from build123d import *
from OCP.BRepFilletAPI import BRepFilletAPI_MakeChamfer

# Parameters (mm, degrees)
ESQUISSE1_W             = 20.32
ESQUISSE1_H             = 13.2
BOSS_EXTRU_1_DEPTH      = 6
ESQUISSE2_W             = 18.32
ESQUISSE2_H             = 11.2
ENL_V_MAT_EXTRU_1_DEPTH = 5
ESQUISSE3_W             = 5
ESQUISSE3_H             = 1
ENL_V_MAT_EXTRU_2_DEPTH = 5
ESQUISSE4_W             = 15.32
ESQUISSE4_H             = 8.2
ENL_V_MAT_EXTRU_3_DEPTH = 25.741511676
ESQUISSE6_W             = 1
ESQUISSE6_H             = 11.2
ENL_V_MAT_EXTRU_4_DEPTH = 4.75
ESQUISSE7_W             = 30
ESQUISSE7_H             = 13.2
BOSS_EXTRU_2_DEPTH      = 1.25
ESQUISSE8_W             = 1.25
ESQUISSE8_H             = 13.2
BOSS_EXTRU_3_DEPTH      = 8
ESQUISSE9_W             = 9.25
ESQUISSE9_H             = 1.25
BOSS_EXTRU_4_DEPTH      = 6
CHANFREIN1_SIZE         = 2
CHANFREIN1_SIZE_2       = 3.464101615
ESQUISSE10_W            = 28.75
ESQUISSE10_H            = 1
BOSS_EXTRU_5_DEPTH      = 2
CHANFREIN2_SIZE         = 2
CHANFREIN2_SIZE2        = 3.464101615
ESQUISSE11_W            = 21
ESQUISSE11_H            = 1.433492253
ENL_V_MAT_EXTRU_5_DEPTH = 2
ESQUISSE12_W            = 0.8
ESQUISSE12_H            = 9.25
ENL_V_MAT_EXTRU_6_DEPTH = 2
CONG_1_R                = 1.5


with BuildPart() as part:
    # Esquisse1 → Boss.-Extru.1 (new body)
    with BuildSketch(Plane.XY):
        with Locations((10.16, 6.6)):
            Rectangle(ESQUISSE1_W, ESQUISSE1_H)
    extrude(amount=BOSS_EXTRU_1_DEPTH)

    # Esquisse2 → Enlèv. mat.-Extru.1 (cut)
    with BuildSketch(Plane.XY.offset(6)):
        with Locations((10.16, 6.6)):
            Rectangle(ESQUISSE2_W, ESQUISSE2_H)
    extrude(amount=-ENL_V_MAT_EXTRU_1_DEPTH, mode=Mode.SUBTRACT)

    # Esquisse3 → Enlèv. mat.-Extru.2 (cut)
    with BuildSketch(Plane.XY.offset(6)):
        with Locations((3.5, 12.7)):
            Rectangle(ESQUISSE3_W, ESQUISSE3_H)
    extrude(amount=-ENL_V_MAT_EXTRU_2_DEPTH, mode=Mode.SUBTRACT)

    # Esquisse4 → Enlèv. mat.-Extru.3 (cut, through all)
    with BuildSketch(Plane.XY.offset(1)):
        with Locations((10.16, 6.6)):
            Rectangle(ESQUISSE4_W, ESQUISSE4_H)
    extrude(amount=-ENL_V_MAT_EXTRU_3_DEPTH, mode=Mode.SUBTRACT)

    # Esquisse6 → Enlèv. mat.-Extru.4 (cut)
    with BuildSketch(Plane.XY.offset(6)):
        with Locations((19.82, 6.6)):
            Rectangle(ESQUISSE6_W, ESQUISSE6_H)
    extrude(amount=-ENL_V_MAT_EXTRU_4_DEPTH, mode=Mode.SUBTRACT)

    # Esquisse7 → Boss.-Extru.2 (add)
    with BuildSketch(Plane(origin=(0, 0, 0), x_dir=(-1, 0, 0), z_dir=(0, 0, -1))):
        with Locations((-35.32, 6.6)):
            Rectangle(ESQUISSE7_W, ESQUISSE7_H)
    extrude(amount=-BOSS_EXTRU_2_DEPTH)

    # Esquisse8 → Boss.-Extru.3 (add)
    with BuildSketch(Plane.XY.offset(1.25)):
        with Locations((49.695, 6.6)):
            Rectangle(ESQUISSE8_W, ESQUISSE8_H)
    extrude(amount=BOSS_EXTRU_3_DEPTH)

    # Esquisse9 → Boss.-Extru.4 (add)
    with BuildSketch(Plane(origin=(50.32, 0, 0), x_dir=(0, 0, -1), z_dir=(1, 0, 0))):
        with Locations((-4.625, 11.375)):
            Rectangle(ESQUISSE9_W, ESQUISSE9_H)
        with Locations((-4.625, 1.825)):
            Rectangle(ESQUISSE9_W, ESQUISSE9_H)
    extrude(amount=BOSS_EXTRU_4_DEPTH)

    # Chanfrein1
    # the kernel refuses this chamfer: 3.464101615, 2 mm, written as the material it adds along each edge
    with BuildSketch(Plane(origin=(50.32, 12, 9.25), x_dir=(0, 1, 0), z_dir=(0, 0, -1))) as chanfrein1_piece_1_section:
        Polygon((CHANFREIN1_SIZE, 0), (0, CHANFREIN1_SIZE_2), (0, 0), align=None)
    chanfrein1_piece_1 = extrude(amount=9.25, mode=Mode.PRIVATE)
    chanfrein1_piece_1 = split(chanfrein1_piece_1, bisect_by=Plane(origin=(50.32, 13.2, 9.25), z_dir=(0, -1, 0)), keep=Keep.TOP, mode=Mode.PRIVATE)
    add(chanfrein1_piece_1)
    with BuildSketch(Plane(origin=(50.32, 1.2, 0), x_dir=(0, -1, 0), z_dir=(0, 0, 1))) as chanfrein1_piece_2_section:
        Polygon((CHANFREIN1_SIZE, 0), (0, CHANFREIN1_SIZE_2), (0, 0), align=None)
    chanfrein1_piece_2 = extrude(amount=9.25, mode=Mode.PRIVATE)
    chanfrein1_piece_2 = split(chanfrein1_piece_2, bisect_by=Plane(origin=(50.32, 0, 0), z_dir=(0, 1, 0)), keep=Keep.TOP, mode=Mode.PRIVATE)
    add(chanfrein1_piece_2)

    # Esquisse10 → Boss.-Extru.5 (add)
    with BuildSketch(Plane.XY.offset(1.25)):
        with Locations((34.695, 12.7)):
            Rectangle(ESQUISSE10_W, ESQUISSE10_H)
        with Locations((34.695, 0.5)):
            Rectangle(ESQUISSE10_W, ESQUISSE10_H)
    extrude(amount=BOSS_EXTRU_5_DEPTH)

    # Chanfrein2: one chamfer whose edges measure the first distance from different faces: ONE call of the kernel's chamfer builder (chamfer() names one face for all edges)
    chanfrein2_edges_1 = [part.edges().sort_by_distance(p)[0] for p in [
        (20.32, 12.7, 3.25),
    ]]
    chanfrein2_side_1 = [part.faces().sort_by_distance(p)[0] for p in [
        (20.32, 12.7, 4.625),
    ]]
    chanfrein2_edges_2 = [part.edges().sort_by_distance(p)[0] for p in [
        (49.07, 12.7, 3.25),
        (49.07, 0.5, 3.25),
    ]]
    chanfrein2_side_2 = [part.faces().sort_by_distance(p)[0] for p in [
        (49.07, 6.6, 5.368110236),
    ]]
    chanfrein2_edges_3 = [part.edges().sort_by_distance(p)[0] for p in [
        (20.32, 0.5, 3.25),
    ]]
    chanfrein2_side_3 = [part.faces().sort_by_distance(p)[0] for p in [
        (20.32, 0.5, 4.625),
    ]]
    chanfrein2 = BRepFilletAPI_MakeChamfer(part.part.solid().wrapped)
    for e in chanfrein2_edges_1:
        chanfrein2.Add(CHANFREIN2_SIZE, CHANFREIN2_SIZE2, e.wrapped, chanfrein2_side_1[0].wrapped)  # the first distance lies on this face
    for e in chanfrein2_edges_2:
        chanfrein2.Add(CHANFREIN2_SIZE, CHANFREIN2_SIZE2, e.wrapped, chanfrein2_side_2[0].wrapped)  # the first distance lies on this face
    for e in chanfrein2_edges_3:
        chanfrein2.Add(CHANFREIN2_SIZE, CHANFREIN2_SIZE2, e.wrapped, chanfrein2_side_3[0].wrapped)  # the first distance lies on this face
    add(Compound.cast(chanfrein2.Shape()), mode=Mode.REPLACE)

    # Esquisse11 → Enlèv. mat.-Extru.5 (cut)
    with BuildSketch(Plane.XY.offset(1.25)):
        with Locations((35.07, 9.983253874)):
            Rectangle(ESQUISSE11_W, ESQUISSE11_H)
        with Locations((35.07, 6.683253873)):
            Rectangle(ESQUISSE11_W, ESQUISSE11_H)
        with Locations((35.07, 3.383253874)):
            Rectangle(ESQUISSE11_W, ESQUISSE11_H)
    extrude(amount=-ENL_V_MAT_EXTRU_5_DEPTH, mode=Mode.SUBTRACT)

    # Esquisse12 → Enlèv. mat.-Extru.6 (cut)
    with BuildSketch(Plane(origin=(0, 1.2, 0), x_dir=(-1, 0, 0), z_dir=(0, -1, 0))):
        with Locations((-55.92, -4.625)):
            Rectangle(ESQUISSE12_W, ESQUISSE12_H)
    extrude(amount=-ENL_V_MAT_EXTRU_6_DEPTH, mode=Mode.SUBTRACT)

    # Congé1
    # the kernel refuses this fillet: 1.5 mm, written as the material it adds along each edge
    with BuildSketch(Plane(origin=(1, 1, 1), x_dir=(0, 0, 1), z_dir=(0, 1, 0))) as cong_1_piece_1:
        with BuildLine():
            CenterArc((CONG_1_R, CONG_1_R), CONG_1_R, 180, 90)
            Line((0, CONG_1_R), (0, 0))
            Line((0, 0), (CONG_1_R, 0))
        make_face()
    extrude(amount=12.2)
    with BuildSketch(Plane(origin=(6, 12.2, 1), x_dir=(-1, 0, 0), z_dir=(0, 1, 0))) as cong_1_piece_2:
        with BuildLine():
            CenterArc((CONG_1_R, CONG_1_R), CONG_1_R, 180, 90)
            Line((0, CONG_1_R), (0, 0))
            Line((0, 0), (CONG_1_R, 0))
        make_face()
    extrude(amount=1)
    # the kernel refuses this fillet: 1.5 mm, written as the material it takes off along each edge
    with BuildSketch(Plane(origin=(20.32, -3.247595264, 6), x_dir=(-1, 0, 0), z_dir=(0, 1, 0)), Plane(origin=(20.32, 8.952404736, 6), x_dir=(-1, 0, 0), z_dir=(0, 1, 0))) as cong_1_2_piece_1:
        with BuildLine():
            CenterArc((1.299038106, -1.5), CONG_1_R, 90, 60)
            Line((0, -0.75), (0, 0))
            Line((0, 0), (1.299038106, 0))
        make_face()
    extrude(amount=7.495190528, mode=Mode.SUBTRACT)
    with BuildSketch(Plane(origin=(19.32, 1, 1.25), x_dir=(1, 0, 0), z_dir=(0, 1, 0))) as cong_1_2_piece_2:
        with BuildLine():
            CenterArc((0.829156198, 1.5), CONG_1_R, 236.442690238, 33.557309762)
            Line((0, 0.25), (0, 0))
            Line((0, 0), (0.829156198, 0))
        make_face()
    extrude(amount=11.2, mode=Mode.SUBTRACT)
    with BuildSketch(Plane(origin=(6, 8.45, 6), x_dir=(0, 0, -1), z_dir=(0, 1, 0))) as cong_1_2_piece_3:
        with BuildLine():
            CenterArc((CONG_1_R, -CONG_1_R), CONG_1_R, 90, 90)
            Line((0, -CONG_1_R), (0, 0))
            Line((0, 0), (CONG_1_R, 0))
        make_face()
    extrude(amount=8.5, mode=Mode.SUBTRACT)


solid = part.part
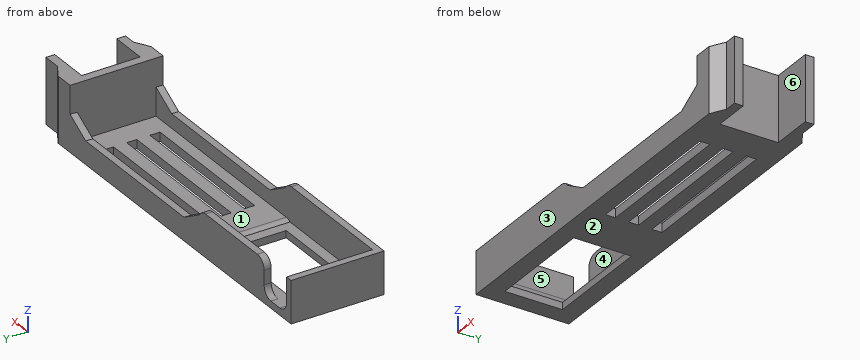
For this review, take the finished solid that the model builds, in its own axes (mm). Face numbers are marked on the shaded views. A direction names the side the tool comes from. Coordinates: 2 decimals unless noted, no trailing zeros. Loops run counter-clockwise (first coordinate to the right, second up) from the corner with the lowest first, then second, coordinate; pieces in that order, holes last. Notation, with made-up numbers: (71.5, 1) -> (121.5, 1) arc R10 ccw to (121.5, 9) -> close; hole circle Ø5 at (85, -12). An arc over 180 degrees is marked (long way). Write each question's results on one line, items separated by ' | '.
Q1. Add section D-D, the plane z = 7.5. State the section outline as (x, y) points, then the cut area to 3 significant figures.
Taken from the geometry:
outline: (49.07, 0) -> (51.71, 0) -> (53.78, 1.2) -> (55.52, 1.2) -> (55.52, 2.45) -> (50.32, 2.45) -> (50.32, 10.75) -> (56.32, 10.75) -> (56.32, 12) -> (53.78, 12) -> (51.71, 13.2) -> (49.07, 13.2) -> close | area: 36.3 mm²
Q2. Machinability: for the marked faces 4, 5 and 6, which of the approach directions +Z, -Z, +X, -X, +Y, -Y give a long, thin tool a straight path to every point of the face, cutting with its end or side? Answer none if there is none.
Taken from the geometry:
face 4: +Z | face 5: +Z, +Y | face 6: +Z, -Z, +X
Q3. For pin 1 Ø2 at (x, y) = (10, 10) entering from -Z; pin 2 Ø1 at (y, z) = (1.5, 4.5) entering from +X; pin 3 Ø3.5 at (x, y) = (35.5, 5) entering from +Z; pin 4 Ø1.1 at (y, z) = (5.5, 0.5) entering from +X, all flat-tipped, find the tip position at first contact; note any pin that passes through.
Taken from the geometry:
pin 1: z = 0 | pin 2: x = 55.52 | pin 3: z = 1.25 | pin 4: x = 50.32
Q4. Add section C-C, the plane z = 0.5. State the section outline as (x, y) points.
Taken from the geometry:
outline: (0, 0) -> (51.71, 0) -> (53.78, 1.2) -> (55.52, 1.2) -> (55.52, 2.45) -> (50.32, 2.45) -> (50.32, 10.75) -> (56.32, 10.75) -> (56.32, 12) -> (53.78, 12) -> (51.71, 13.2) -> (0, 13.2) -> close; hole (2.5, 2.5) -> (17.82, 2.5) -> (17.82, 10.7) -> (2.5, 10.7) -> close; hole (24.57, 2.67) -> (45.57, 2.67) -> (45.57, 4.1) -> (24.57, 4.1) -> close; hole (24.57, 5.97) -> (45.57, 5.97) -> (45.57, 7.4) -> (24.57, 7.4) -> close; hole (24.57, 9.27) -> (45.57, 9.27) -> (45.57, 10.7) -> (24.57, 10.7) -> close
Q5. Add section A-A, the plane x = 33. State the section outline as (y, z) points, then the cut area to 3 significant figures.
Taken from the geometry:
outline: (0, 0) -> (2.67, 0) -> (2.67, 1.25) -> (1, 1.25) -> (1, 3.25) -> (0, 3.25) -> close; (4.1, 0) -> (5.97, 0) -> (5.97, 1.25) -> (4.1, 1.25) -> close; (7.4, 0) -> (9.27, 0) -> (9.27, 1.25) -> (7.4, 1.25) -> close; (10.7, 0) -> (13.2, 0) -> (13.2, 3.25) -> (12.2, 3.25) -> (12.2, 1.25) -> (10.7, 1.25) -> close | area: 15.1 mm²
Q6. To check wall thickness, follow line 1 along Y through (x, z) = (6, 1.5); line 2 along Y through (x, z) = (50.5, 4); line 3 along X through (y, z) = (5.25, 4.75). State the ranges of each line that lie inside material, in increasing order. Write a range as [from, to].
Taken from the geometry:
line 1: [0, 1], [12.2, 13.2] | line 2: [0, 2.45], [10.75, 13.2] | line 3: [0, 1], [49.07, 50.32]
Q7. Add section B-B, the plane y = 6.75. State the section outline as (x, z) points.
Taken from the geometry:
outline: (0, 0) -> (2.5, 0) -> (2.5, 1) arc R1.5 cw to (1, 2.5) -> (1, 6) -> (0, 6) -> close; (17.82, 0) -> (24.57, 0) -> (24.57, 1.25) -> (20.15, 1.25) arc R1.5 ccw to (19.32, 1) -> (17.82, 1) -> close; (45.57, 0) -> (50.32, 0) -> (50.32, 9.25) -> (49.07, 9.25) -> (49.07, 1.25) -> (45.57, 1.25) -> close
Q8. Mouldability with a two-part tool opening along Y and no side actions: class the marked faces 1, 2 and 3 as +Y half, -Y half, draft (parallel to the pull), parting line (faces both ways), or undercut.
Taken from the geometry:
face 1: undercut | face 2: draft | face 3: -Y half
